```python
from build123d import *

# Parameters (mm, degrees)
SKETCH1_W               = 101.6
SKETCH1_H               = 76.2
BOSS_EXTRUDE1_DEPTH     = 25.4
SKETCH5_W               = 91.44
SKETCH5_H               = 71.12
CUT_EXTRUDE1_DEPTH      = 20.32
FILLET1_R               = 2.54
SKETCH7_W               = 2.54
SKETCH7_H               = 2.54
BOSS_EXTRUDE2_DEPTH     = 6.35
BOSS_EXTRUDE2_TAPER     = 1
MIRROR4_COPY_1_SKETCH_W = 2.54
MIRROR4_COPY_1_SKETCH_H = 2.54
MIRROR4_COPY_1_DEPTH    = 6.35
MIRROR4_COPY_1_TAPER    = 1
SKETCH8_W               = 60.96
SKETCH8_H               = 12.7
CUT_EXTRUDE2_DEPTH      = 71.99515833
SKETCH9_W               = 50.8
SKETCH9_H               = 20.32
BOSS_EXTRUDE3_DEPTH     = 2.54


with BuildPart() as part:
    # Sketch1 → Boss-Extrude1 (new body)
    with BuildSketch(Plane(origin=(0, 0, 0), x_dir=(1, 0, 0), z_dir=(0, 1, 0))):
        Rectangle(SKETCH1_W, SKETCH1_H)
    extrude(amount=BOSS_EXTRUDE1_DEPTH)

    # Sketch5 → Cut-Extrude1 (cut)
    with BuildSketch(Plane.XZ):
        Rectangle(SKETCH5_W, SKETCH5_H)
    extrude(amount=-CUT_EXTRUDE1_DEPTH, mode=Mode.SUBTRACT)

    # Fillet1
    fillet1_edges = [part.edges().sort_by_distance(p)[0] for p in [
        (-50.8, 25.4, 0),
        (0, 25.4, 38.1),
        (50.8, 25.4, 0),
        (50.8, 12.7, 38.1),
        (-50.8, 12.7, 38.1),
        (-50.8, 12.7, -38.1),
        (50.8, 12.7, -38.1),
        (0, 25.4, -38.1),
    ]]
    fillet(fillet1_edges, radius=FILLET1_R)

    # Sketch7 → Boss-Extrude2 (add)
    with BuildSketch(Plane(origin=(0, 0, 0), x_dir=(-1, 0, 0), z_dir=(0, -1, 0))):
        with Locations((48.26, -35.56)):
            Rectangle(SKETCH7_W, SKETCH7_H)
    boss_extrude2 = extrude(amount=BOSS_EXTRUDE2_DEPTH, taper=BOSS_EXTRUDE2_TAPER)

    # Mirror3: Boss-Extrude2 across plane
    add(boss_extrude2.mirror(Plane(origin=(0, 0, 0), x_dir=(0, 0, 1), z_dir=(1, 0, 0))))

    # Mirror4: Boss-Extrude2 across plane
    add(boss_extrude2.mirror(Plane.XY))

    # Mirror4 copy 1 sketch → Mirror4 copy 1 (add)
    with BuildSketch(Plane.XZ):
        with Locations((48.26, -35.56)):
            Rectangle(MIRROR4_COPY_1_SKETCH_W, MIRROR4_COPY_1_SKETCH_H)
    extrude(amount=MIRROR4_COPY_1_DEPTH, taper=MIRROR4_COPY_1_TAPER)

    # Sketch8 → Cut-Extrude2 (cut, through all)
    with BuildSketch(Plane(origin=(0, 25.4, 0), x_dir=(1, 0, 0), z_dir=(0, 1, 0))):
        with Locations((0, -25.4)):
            Rectangle(SKETCH8_W, SKETCH8_H)
    extrude(amount=-CUT_EXTRUDE2_DEPTH, mode=Mode.SUBTRACT)

    # Sketch9 → Boss-Extrude3 (add)
    with BuildSketch(Plane(origin=(0, 0, 35.56), x_dir=(-1, 0, 0), z_dir=(0, 0, -1))):
        with Locations((0, 10.16)):
            Rectangle(SKETCH9_W, SKETCH9_H)
    extrude(amount=BOSS_EXTRUDE3_DEPTH)


solid = part.part
```
Part model, mm, in its own coordinate system. A direction names the side the tool comes from. Coordinates: 2 decimals unless noted, no trailing zeros. Order: outer loops, then holes, each group sorted by start corner. A loop starts at its lowest first (then second) coordinate and runs counter-clockwise, first axis right, second up. Notation, with made-up numbers: (13, -31) - (64, -31) arc R12 cw to (64, -27) - close; hole circle Ø10 at (-10, 78.5). An arc over 180 degrees is marked (long way). Return JSON: item names as keys, results as strings. Group by question number.
Item 1: Cut at B-B (x = 3.5). List the corners of the cut face in (y, z), plus the area to 3 significant figures.
Item 2: Cut at D-D (y = -4). State how many separate pieces and enclosed holes the cut face has, plus the area to 3 significant figures.
Item 3: Drill centre lines: probe 1 along X at (y, z) = (10, 31); probe 2 along Z at (x, y) = (-22.5, 20.5); probe 3 along Z at (x, y) = (-30, 10). Where is each one in solid material? Low to high. Write a range as from..to.
Item 4: Pin check, flat tips, straight feed: pin 1 (1 mm diameter, centred on x = -37, z = 28, fed in from -Y); pin 2 (1.5 mm diameter, centred on y = 23.5, z = 26, fed in from -X); pin 3 (1.5 mm diameter, centred on x = 5, y = 24, fed in from +Z). Stop position of each tip, or through.
Item 5: Pull direction Z, two halves, no side cores. Call faces 4 (the face through (-1, 11, -38.1)), 5 (the face through (35, 10, 35.56)), 6 (the face through (-48, -6.35, -36)), 7 (the face through (25.4, 10, 34)): pulls with the +Z half, pulls with the -Z half, needs draft (parallel to the pull), parting line crosses it, or undercut.
Item 6: Cut at A-A (y = 9.5). List the corners of the cut face in (x, z), plus the area to 3 significant figures.
Item 7: Cut at C-C (z = 7). List the corners of the cut face in (x, y).
Item 8: Which spindle directions (+Z, -Z, +X, -X, +Y, -Y) get a long thin tool onto all of the face, cutting with end or side? Do faces 1 (the face through (-1, 25.4, 0)), 2 (the face through (0, 23, 31.75)), 3 (the face through (-1, 10, -35.56)). Say none if no direction does.
Check values:
{
 "1": {"outline": "(0, -38.1) - (22.86, -38.1) arc R2.54 ccw to (25.4, -35.56) - (25.4, 19.05) - (20.32, 19.05) - (20.32, -35.56) - (0, -35.56) - close; (0, 33.02) - (20.32, 33.02) - (20.32, 31.75) - (25.4, 31.75) - (25.4, 35.56) arc R2.54 ccw to (22.86, 38.1) - (0, 38.1) - close", "area": "475 mm2"},
 "2": {"separate pieces": "4", "enclosed holes": "0", "area": "23.0 mm2"},
 "3": {"probe 1": "x = -50.8..-45.72, 45.72..50.8", "probe 2": "z = -38.1..19.05, 31.75..38.1", "probe 3": "z = -38.1..-35.56, 35.56..38.1"},
 "4": {"pin 1": "stops at y = 20.32", "pin 2": "stops at x = -50.8", "pin 3": "stops at z = 38.07"},
 "5": {"face 4": "pulls with the -Z half", "face 5": "undercut", "face 6": "needs draft", "face 7": "undercut"},
 "6": {"outline": "(-50.8, -35.56) arc R2.54 ccw to (-48.26, -38.1) - (48.26, -38.1) arc R2.54 ccw to (50.8, -35.56) - (50.8, 35.56) arc R2.54 ccw to (48.26, 38.1) - (-48.26, 38.1) arc R2.54 ccw to (-50.8, 35.56) - close; hole (-45.72, -35.56) - (45.72, -35.56) - (45.72, 35.56) - (25.4, 35.56) - (25.4, 33.02) - (-25.4, 33.02) - (-25.4, 35.56) - (-45.72, 35.56) - close", "area": "1,360 mm2"},
 "7": {"outline": "(-50.8, 0) - (-45.72, 0) - (-45.72, 20.32) - (45.72, 20.32) - (45.72, 0) - (50.8, 0) - (50.8, 22.86) arc R2.54 ccw to (48.26, 25.4) - (-48.26, 25.4) arc R2.54 ccw to (-50.8, 22.86) - close"},
 "8": {"face 1": "+Z, -Z, +X, -X, +Y", "face 2": "+Y, -Y", "face 3": "-Y"}
}
